Could you check a few things on this drawing? It's one solid part, dimensions in mm from its lowest x, y, z. A direction names the side the tool comes from. Round coordinates to 2 decimals unless told otherwise and drop trailing zeros. Loops run counter-clockwise (first coordinate to the right, second up) from the corner with the lowest first, then second, coordinate; pieces in that order, holes last. Notation, with made-up numbers: M 71,6 L 78,6 A11 ccw 78,10 Z; hole C 12,-12 d8. An arc over 180 degrees is marked long. Return JSON: item names as keys, results as strings.
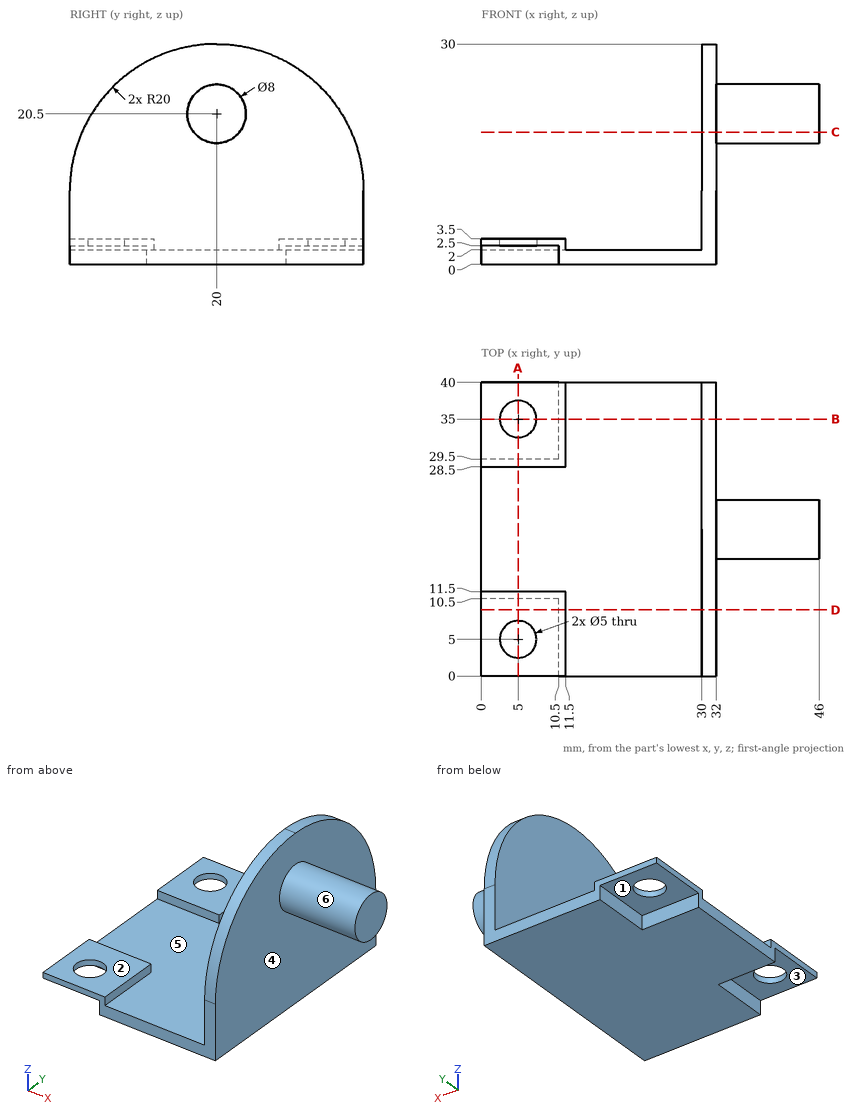
Q1. Suppose I cut it at B-B, the plane y = 35. Please give me the cut outline in (x, z).
Results:
{"outline": "M 0,2.5 L 2.5,2.5 L 2.5,3.5 L 0,3.5 Z; M 7.5,2.5 L 10.5,2.5 L 10.5,0 L 32,0 L 32,23.23 L 30,23.23 L 30,2 L 11.5,2 L 11.5,3.5 L 7.5,3.5 Z"}
Q2. Suppose I cut it at A-A, the plane x = 5. Please give me the cut outline in (y, z).
Results:
{"outline": "M 0,2.5 L 2.5,2.5 L 2.5,3.5 L 0,3.5 Z; M 7.5,2.5 L 10.5,2.5 L 10.5,0 L 29.5,0 L 29.5,2.5 L 32.5,2.5 L 32.5,3.5 L 28.5,3.5 L 28.5,2 L 11.5,2 L 11.5,3.5 L 7.5,3.5 Z; M 37.5,2.5 L 40,2.5 L 40,3.5 L 37.5,3.5 Z"}
Q3. Suppose I cut it at C-C, the plane z = 18. Please give me the cut outline in (x, y).
Results:
{"outline": "M 30,1.67 L 32,1.67 L 32,16.88 L 46,16.88 L 46,23.12 L 32,23.12 L 32,38.33 L 30,38.33 Z"}
Q4. If I drill on line 1 along Y through (x, z) = (5, 3); line 2 along Z through (x, y) = (12.5, 38); line 3 along X through (y, z) = (21, 28.5), over which ranges is the centre line in solid material (lowest first)?
Results:
{"line 1": "y = 0 to 2.5, 7.5 to 11.5, 28.5 to 32.5, 37.5 to 40", "line 2": "z = 0 to 2", "line 3": "x = 30 to 32"}
Q5. On a 3-axis mill with a long thin cutter (end or side, diameter ignored), from which of +Z, -Z, +X, -X, +Y, -Y can I reach the whole of each face in a straight line? I mean the marked faces 1, 2 and 3. Say none if no direction works.
Results:
{"face 1": "-Z, -X, +Y", "face 2": "+Z, -X, +Y, -Y", "face 3": "-Z, -X, -Y"}
Q6. Thinking about a two-plate mould opening in X: for the marked faces 4, 5 and 6, which applies, pulls with the +X half, pulls with the -X half, needs draft (parallel to the pull), parting line crosses it, or undercut?
Results:
{"face 4": "pulls with the +X half", "face 5": "undercut", "face 6": "needs draft"}
Q7. Suppose I cut it at D-D, the plane y = 9. Please give me the cut outline in (x, z), plus the area to 3 significant figures.
Results:
{"outline": "M 0,2.5 L 10.5,2.5 L 10.5,0 L 32,0 L 32,26.7 L 30,26.7 L 30,2 L 11.5,2 L 11.5,3.5 L 0,3.5 Z", "area": "104 mm2"}
Q8. I'm going to push flat-ended pins straight in: pin 1 Ø5 at (y, z) = (22, 25.5) entering from -X; pin 2 Ø6 at (x, y) = (31, 8) entering from +Z; pin 3 Ø9 at (x, y) = (4.5, 8.5) entering from +Z. Where does each tip first touch, or does it pass through?
Results:
{"pin 1": "stops at x = 30", "pin 2": "stops at z = 27.86", "pin 3": "stops at z = 3.5"}
